Autodesk Inventor part; units mm, degrees
ref_plane "YZ Plane" through (0, 0, 0) normal (1, 0, 0) x (0, 1, 0)
ref_plane "XZ Plane" through (0, 0, 0) normal (0, 1, 0) x (-1, 0, 0)
ref_plane "XY Plane" through (0, 0, 0) normal (0, 0, 1) x (1, 0, 0)
sketch "Sketch1" plane through (0, 0, 0) normal (0, 1, 0) x (-1, 0, 0)
  line L0 (0, 0) -> (80, 0)
  line L1 (80, 0) -> (80, -400)
  line L2 (80, -400) -> (0, -400)
  line L3 (0, -400) -> (0, 0)
  line L4 (76, -4) -> (42, -4)
  line L5 (42, -4) -> (42, -39.6)
  line L6 (42, -39.6) -> (76, -39.6)
  line L7 (76, -39.6) -> (76, -4)
  line L8 (76, -43.6) -> (42, -43.6)
  line L9 (42, -43.6) -> (42, -79.2)
  line L10 (42, -79.2) -> (76, -79.2)
  line L11 (76, -79.2) -> (76, -43.6)
  line L12 (76, -83.2) -> (42, -83.2)
  line L13 (42, -83.2) -> (42, -118.8)
  line L14 (42, -118.8) -> (76, -118.8)
  line L15 (76, -118.8) -> (76, -83.2)
  line L16 (76, -122.8) -> (42, -122.8)
  line L17 (42, -122.8) -> (42, -158.4)
  line L18 (42, -158.4) -> (76, -158.4)
  line L19 (76, -158.4) -> (76, -122.8)
  line L20 (76, -162.4) -> (42, -162.4)
  line L21 (42, -162.4) -> (42, -198)
  line L22 (42, -198) -> (76, -198)
  line L23 (76, -198) -> (76, -162.4)
  line L24 (76, -202) -> (42, -202)
  line L25 (42, -202) -> (42, -237.6)
  line L26 (42, -237.6) -> (76, -237.6)
  line L27 (76, -237.6) -> (76, -202)
  line L28 (76, -241.6) -> (42, -241.6)
  line L29 (42, -241.6) -> (42, -277.2)
  line L30 (42, -277.2) -> (76, -277.2)
  line L31 (76, -277.2) -> (76, -241.6)
  line L32 (76, -281.2) -> (42, -281.2)
  line L33 (42, -281.2) -> (42, -316.8)
  line L34 (42, -316.8) -> (76, -316.8)
  line L35 (76, -316.8) -> (76, -281.2)
  line L36 (76, -320.8) -> (42, -320.8)
  line L37 (42, -320.8) -> (42, -356.4)
  line L38 (42, -356.4) -> (76, -356.4)
  line L39 (76, -356.4) -> (76, -320.8)
  line L40 (38, -4) -> (4, -4)
  line L41 (4, -4) -> (4, -39.6)
  line L42 (4, -39.6) -> (38, -39.6)
  line L43 (38, -39.6) -> (38, -4)
  line L44 (38, -43.6) -> (4, -43.6)
  line L45 (4, -43.6) -> (4, -79.2)
  line L46 (4, -79.2) -> (38, -79.2)
  line L47 (38, -79.2) -> (38, -43.6)
  line L48 (38, -83.2) -> (4, -83.2)
  line L49 (4, -83.2) -> (4, -118.8)
  line L50 (4, -118.8) -> (38, -118.8)
  line L51 (38, -118.8) -> (38, -83.2)
  line L52 (38, -122.8) -> (4, -122.8)
  line L53 (4, -122.8) -> (4, -158.4)
  line L54 (4, -158.4) -> (38, -158.4)
  line L55 (38, -158.4) -> (38, -122.8)
  line L56 (38, -162.4) -> (4, -162.4)
  line L57 (4, -162.4) -> (4, -198)
  line L58 (4, -198) -> (38, -198)
  line L59 (38, -198) -> (38, -162.4)
  line L60 (38, -202) -> (4, -202)
  line L61 (4, -202) -> (4, -237.6)
  line L62 (4, -237.6) -> (38, -237.6)
  line L63 (38, -237.6) -> (38, -202)
  line L64 (38, -241.6) -> (4, -241.6)
  line L65 (4, -241.6) -> (4, -277.2)
  line L66 (4, -277.2) -> (38, -277.2)
  line L67 (38, -277.2) -> (38, -241.6)
  line L68 (38, -281.2) -> (4, -281.2)
  line L69 (4, -281.2) -> (4, -316.8)
  line L70 (4, -316.8) -> (38, -316.8)
  line L71 (38, -316.8) -> (38, -281.2)
  line L72 (38, -320.8) -> (4, -320.8)
  line L73 (4, -320.8) -> (4, -356.4)
  line L74 (4, -356.4) -> (38, -356.4)
  line L75 (38, -356.4) -> (38, -320.8)
  line L76 (76, -360.4) -> (4, -360.4)
  line L77 (4, -360.4) -> (4, -396)
  line L78 (4, -396) -> (76, -396)
  line L79 (76, -396) -> (76, -360.4)
  dimension "d0" = 80
  dimension "d1" = 400
  dimension "d2" = 4
  dimension "d3" = 4
  dimension "d4" = 34
  dimension "d5" = 35.6
  dimension "d8" = 39.6
  dimension "d11" = 38
  dimension "d14" = 4
  dimension "d15" = 4
  dimension "d16" = 4
  dimension "d17" = 4
extrude "Extrusion1" add sketch "Sketch1" along normal blind 60
sketch "Sketch2" plane through (0, 60, 0) normal (0, 1, 0) x (1, 0, 0)
  line L0 (-80, 0) -> (0, 0)
  line L1 (0, 400) -> (-80, 400)
  line L2 (-80, 0) -> (0, 0)
  line L3 (0, 0) -> (0, 400)
  line L4 (0, 400) -> (-80, 400)
  line L5 (-80, 400) -> (-80, 0)
extrude "Extrusion2" add sketch "Sketch2" along normal blind 4
properties part number "Contenedor Sólido" material "ABS Plastic"
The model under review builds one solid part; all positions refer to its coordinate system, in mm. A direction names the side the tool comes from. Give positions to 0.01 mm unless a question says otherwise; leave off trailing zeros. Write each loop counter-clockwise with the first axis right and the second up, starting at its lowest first coordinate (ties: lowest second). Pieces come first, ordered by that corner, then holes. Notation, with made-up numbers: M 76.5,13.5 L 122.5,13.5 A13 ccw 122.5,19.5 Z; hole C 44,9 d10. An arc over 180 degrees is marked long. Write item = value, one per line. Start each with the question number.
Q1. We need section C-C (z = -104). State the section outline as (x, y) points, plus the area to 3 significant figures.
Q2. Machinability: for faces 1 (the face through (-40, 0, -199)), 2 (the face through (-21, 30, -202)), which of the approach directions +Z, -Z, +X, -X, +Y, -Y give a long, thin tool a straight path to every point of the face, cutting with its end or side? Answer none if there is none.
Q3. For line 1 (X direction, y = 42.5, z = -78); line 2 (Z direction, x = -40, y = 49); line 3 (Y direction, x = -57, z = -274), list the stretches that pass through material, from the lowest coordinate up.
Q4. We need section B-B (y = 9.5). Give the number of separate pieces and of enclosed holes in the cut face, plus the area to 3 significant figures.
Q5. Clearance check with a flat-ended pin moving along its axis: pin 1 (17 mm diameter, centred on x = -23.5, z = -15, fed in from -Y). State where the tip first meets the part, or that it passes through.
Q6. Mouldability with a two-part tool opening along X and no side actions: class faces 3 (the face through (-42, 30, -338)), 4 (the face through (-39, 32, 0)), 5 (the face through (-76, 30, -62)) as released by +X, released by -X, zero draft, split by the parting line, or undercut.
Q7. We need section A-A (z = -370). State the section outline as (x, y) points.
Result set:
q1.outline = M -80,0 L -76,0 L -76,60 L -42,60 L -42,0 L -38,0 L -38,60 L -4,60 L -4,0 L 0,0 L 0,64 L -80,64 Z
q1.area = 1,040 mm2
q2.face_1 = +Z, -Z, +X, -X, -Y
q2.face_2 = -Y
q3.line_1 = -80 to -76, -42 to -38, -4 to 0
q3.line_2 = -400 to -396, -360.4 to 0
q3.line_3 = 60 to 64
q4.separate_pieces = 1
q4.enclosed_holes = 19
q4.area = 7,650 mm2
q5.pin_1 = 60
q6.face_3 = undercut
q6.face_4 = zero draft
q6.face_5 = undercut
q7.outline = M -80,0 L -76,0 L -76,60 L -4,60 L -4,0 L 0,0 L 0,64 L -80,64 Z
